from build123d import *

# Parameters (mm, degrees)
BOSS_EXTRUDE3_DEPTH = 8


with BuildPart() as part:
    # Sketch1 → Boss-Extrude3 (new body)
    with BuildSketch(Plane.XY):
        with BuildLine():
            Line((-245, -2.75), (-245, -72.5))
            Line((-245, -72.5), (-2.75, -72.5))
            Line((-2.75, -72.5), (-2.75, -47.5))
            ThreePointArc((-2.75, -47.5), (0, -44.75), (2.75, -47.5))
            Line((2.75, -47.5), (2.75, -72.5))
            Line((2.75, -72.5), (245, -72.5))
            Line((245, -72.5), (245, -2.75))
            Line((245, -2.75), (220, -2.75))
            ThreePointArc((220, -2.75), (217.25, 0), (220, 2.75))
            Line((220, 2.75), (245, 2.75))
            Line((245, 2.75), (245, 72.5))
            Line((245, 72.5), (2.75, 72.5))
            Line((2.75, 72.5), (2.75, 47.5))
            ThreePointArc((2.75, 47.5), (0, 44.75), (-2.75, 47.5))
            Line((-2.75, 47.5), (-2.75, 72.5))
            Line((-2.75, 72.5), (-245, 72.5))
            Line((-245, 72.5), (-245, 2.75))
            Line((-245, 2.75), (-220, 2.75))
            ThreePointArc((-220, 2.75), (-217.25, 0), (-220, -2.75))
            Line((-220, -2.75), (-245, -2.75))
        make_face()
        with BuildLine():
            ThreePointArc((-45, -15), (-60, 0), (-45, 15))
            Line((-45, 15), (45, 15))
            ThreePointArc((45, 15), (60, 0), (45, -15))
            Line((45, -15), (-45, -15))
        make_face(mode=Mode.SUBTRACT)
    extrude(amount=BOSS_EXTRUDE3_DEPTH)


solid = part.part
Can you work these out from the model? Positions are in its coordinate system, mm. A direction names the side the tool comes from. Coordinates: 2 decimals unless noted, no trailing zeros. Order: outer loops, then holes, each group sorted by start corner. A loop starts at its lowest first (then second) coordinate and runs counter-clockwise, first axis right, second up. Notation, with made-up numbers: M 53.5,74.5 L 105.5,74.5 A28 cw 105.5,111.5 Z; hole C 20.5,77 d9. An arc over 180 degrees is marked long. Write item = value, one per line.
(1) If we mould it in two halves opening along Y, with no side actions, what happens to faces 1 (the face through (126, 72.5, 4)), 2 (the face through (232, 2.75, 4)), 3 (the face through (122, -72.5, 4)), 4 (the face through (245, -38, 4))? For each: pulls with the +Y half, pulls with the -Y half, needs draft (parallel to the pull), parting line crosses it, or undercut.
Results are:
face_1 = pulls with the +Y half
face_2 = undercut
face_3 = pulls with the -Y half
face_4 = needs draft
(2) I need wall thicknesses on line 1 along X through (y, z) = (-63, 6.25); line 2 along Y through (x, z) = (-36, 6.5); line 3 along X through (y, z) = (-4.5, 7). Which ranges of each line are inside material? Lowest first, please. Write a range as [from, to].
Results are:
line_1 = [-245, -2.75], [2.75, 245]
line_2 = [-72.5, -15], [15, 72.5]
line_3 = [-245, -59.31], [59.31, 245]
(3) Suppose I cut it at A-A on z = 5.5. Please give me the cut outline in (x, y).
Results are:
outline = M -245,-72.5 L -2.75,-72.5 L -2.75,-47.5 A2.75 cw 2.75,-47.5 L 2.75,-72.5 L 245,-72.5 L 245,-2.75 L 220,-2.75 A2.75 cw 220,2.75 L 245,2.75 L 245,72.5 L 2.75,72.5 L 2.75,47.5 A2.75 cw -2.75,47.5 L -2.75,72.5 L -245,72.5 L -245,2.75 L -220,2.75 A2.75 cw -220,-2.75 L -245,-2.75 Z; hole M -45,-15 L 45,-15 A15 ccw 45,15 L -45,15 A15 ccw Z
(4) For faces 5 (the face through (233, -2.75, 4)), 6 (the face through (2.75, -60, 4)), 7 (the face through (1, -15, 4)), 8 (the face through (2.75, 60, 4)), which set-ups out of +Z, -Z, +X, -X, +Y, -Y let a thin tool reach every point of the face, with its end or its side?
Results are:
face_5 = +Z, -Z, +X
face_6 = +Z, -Z, -Y
face_7 = +Z, -Z
face_8 = +Z, -Z, +Y
(5) For pin 1 Ø10 at (x, y) = (26, 20) entering from -Z, with a flat end and sliding along its axis, tell me the tip position at first contact or that it passes through.
Results are:
pin_1 = 0
